Source: three-view drawing plus pictorial views. Frame: mm from the lowest corner of the part. A direction names the side the tool comes from. Coordinates: 2 decimals unless noted, no trailing zeros. Write each loop counter-clockwise with the first axis right and the second up, starting at its lowest first coordinate (ties: lowest second). Pieces come first, ordered by that corner, then holes. Notation, with made-up numbers: (42.5, 69.25) - (74.5, 69.25) arc R16 ccw to (74.5, 99.25) - close; hole circle Ø11 at (36.25, 50). An arc over 180 degrees is marked (long way). One line per item, written item: value.
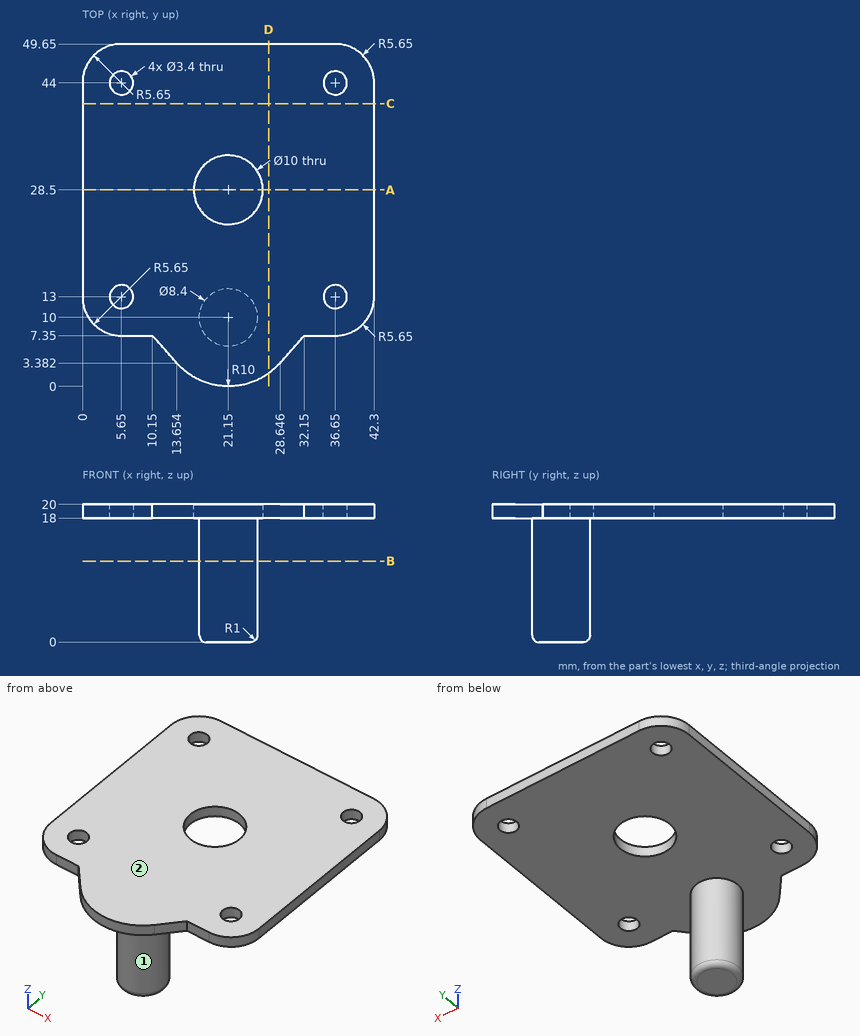
1) Section query D-D on x = 27. Output: boundary loops of the cut face in (y, z).
Values found:
outline: (1.89, 18) - (49.65, 18) - (49.65, 20) - (1.89, 20) - close
2) Material intervals for line 1 (Y direction, x = 36.65, z = 18.5); line 2 (Y direction, x = 21.15, z = 18.5), sorted ascending.
Values found:
line 1: 7.35 to 11.3, 14.7 to 42.3, 45.7 to 49.65
line 2: 0 to 23.5, 33.5 to 49.65
3) Section query C-C on y = 41. Output: boundary loops of the cut face in (x, z).
Values found:
outline: (0, 18) - (42.3, 18) - (42.3, 20) - (0, 20) - close
4) Contact query for flat-ended pins moving along their axis: P1, Ø1.5, axis at x = 8.5, z = 17, coming from the -Y side; P2, Ø2, axis at x = 34, z = 19, coming from the -Y side; P3, Ø3, axis at x = 27.5, y = 17.5, coming from the -Z side; P4, Ø1.5, axis at x = 18, z = 12.5, coming from the -Y side. Output: stop coordinate, or through.
Values found:
P1: through
P2: y = 7.35
P3: z = 18
P4: y = 6.55
5) Reachability of the marked faces 1 and 2 from +Z, -Z, +X, -X, +Y, -Y: full face, straight path, thin tool, end or side. Return the list, or none.
Values found:
face 1: -Z
face 2: +Z, +X, -X, +Y, -Y
6) Section query B-B on z = 11.75. Output: boundary loops of the cut face in (x, y), then the cut area to 3 significant figures.
Values found:
outline: circle Ø8.4 at (21.15, 10)
area: 55.4 mm2
7) Section query A-A on y = 28.5. Output: boundary loops of the cut face in (x, z).
Values found:
outline: (0, 18) - (16.15, 18) - (16.15, 20) - (0, 20) - close; (26.15, 18) - (42.3, 18) - (42.3, 20) - (26.15, 20) - close
